Job drawing, mm, ordinate dimensions from the low corner. One solid piece. A direction names the side the tool comes from. Round coordinates to 2 decimals unless told otherwise and drop trailing zeros. Loops run counter-clockwise (first coordinate to the right, second up) from the corner with the lowest first, then second, coordinate; pieces in that order, holes last. Notation, with made-up numbers: M 28.25,37 L 71.25,37 A19 ccw 71.25,65 Z; hole C 39.25,41 d10. An arc over 180 degrees is marked long. Use a Markdown table: item, result. Add a question column.
(1) Band-saw the part on B-B, the plane y = 29. Write the cut outline in (x, z), and give its area (3 significant figures).
(2) Band-saw the part on D-D, the plane x = 22. Write the cut outline in (y, z), and give its area (3 significant figures).
(3) Flat gauge pins, fed straight in: P1, Ø10, axis at y = 27, z = 16, coming from the +X side; P2, Ø8, axis at x = 39, z = 19, coming from the +Y side. Where does each tip first touch, or does it go through?
(4) Which spindle directions (+Z, -Z, +X, -X, +Y, -Y) get a long thin tool onto all of the face, cutting with end or side? Do the marked faces 1 and 2. Say none if no direction does.
(5) Band-saw the part on A-A, the plane z = 17. Write the cut outline in (x, y).
(6) Band-saw the part on C-C, the plane z = 10. Write the cut outline in (x, y).
(7) Wall check: L1, parallel to Y at x = 20, z = 14. Give the ranges that are in metal, low to high.
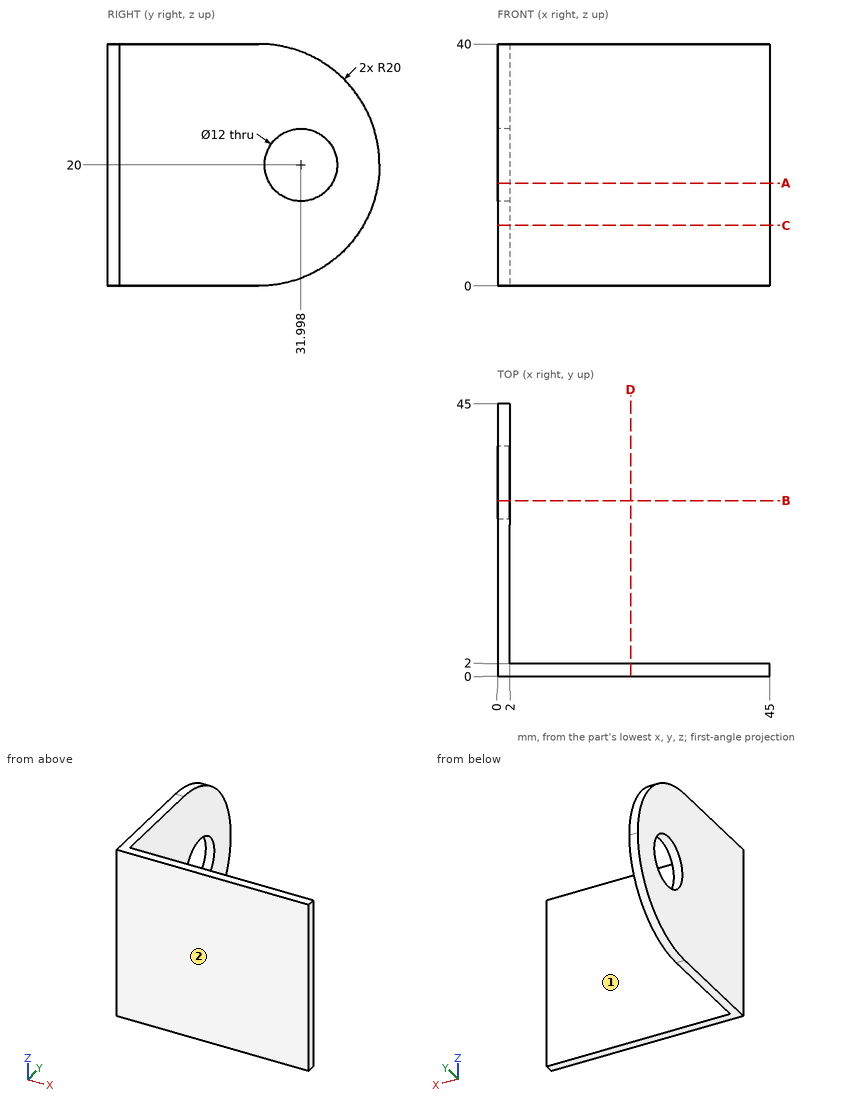
Return value:
| question | item | result |
|---|---|---|
| 1 | outline | M 0,0.4 L 2,0.4 L 2,14.8 L 0,14.8 Z; M 0,25.2 L 2,25.2 L 2,39.6 L 0,39.6 Z |
| 1 | area | 57.6 mm^2 |
| 2 | outline | M 0,0 L 2,0 L 2,40 L 0,40 Z |
| 2 | area | 80.0 mm^2 |
| 3 | P1 | x = 2 |
| 3 | P2 | y = 2 |
| 4 | face 1 | +Z, -Z, +X, +Y |
| 4 | face 2 | +Z, -Z, +X, -X, -Y |
| 5 | outline | M 0,0 L 45,0 L 45,2 L 2,2 L 2,26.8 L 0,26.8 Z; M 0,37.19 L 2,37.19 L 2,44.77 L 0,44.77 Z |
| 6 | outline | M 0,0 L 45,0 L 45,2 L 2,2 L 2,42.32 L 0,42.32 Z |
| 7 | L1 | 0 to 2 |
